Work out the finished part from the listing and answer in its coordinate system (mm). Face numbers are marked on the shaded views. A direction names the side the tool comes from. Round coordinates to 2 decimals unless told otherwise and drop trailing zeros. Order: outer loops, then holes, each group sorted by start corner. A loop starts at its lowest first (then second) coordinate and runs counter-clockwise, first axis right, second up. Notation, with made-up numbers: (89, -5.5) -> (114, -5.5) arc R20 cw to (114, 21.5) -> close; hole circle Ø9 at (-1, 7.25). An arc over 180 degrees is marked (long way). Use a Markdown table: item, result. Add a question column.
Item 1: Flat-ended cylindrical pins translate along their axes: P1, Ø5, axis at x = 77.5, y = -2, coming from the +Z side; P2, Ø20.5, axis at y = -24.5, z = 54.5, coming from the -X side; P3, Ø1.5, axis at y = -11.5, z = 29.5, coming from the +X side (3 decimals); P4, Ø2, axis at x = -40, y = 58.5, coming from the -Z side. Find the tip coordinate at first contact, or state that the pin passes through.
Item 2: A tool of negligible diameter and unlimited length cuts with its end or side. For the marked faces 1, 2, 3 and 4, from which of +Z, -Z, +X, -X, +Y, -Y can it reach the whole face along a straight path? Write none if from no direction.
Item 3: A cutting plane is placed at A-A, the plane x = 0. Determine the outline of the cut face in (y, z) (3 decimals).
Item 4: A cutting plane is placed at B-B, the plane z = 15. Determine the outline of the cut face in (x, y) (3 decimals).
Item 5: A cutting plane is placed at C-C, the plane y = 0. Determine the outline of the cut face in (x, z) (3 decimals), plus the area to 3 significant figures.
Item 6: For a pull along Y with two mould halves and no side action, classify the marked faces 5, 6, 7 and 8 as +Y half, -Y half, draft (parallel to the pull), parting line (faces both ways), or undercut.
Item 7: Find the intervals of material crossed by L1, parallel to Y at x = 0, z = 14 (3 decimals); L2, parallel to X at y = -3, z = 58; L3, parallel to Y at x = 115, z = 11, in increasing order. Write a range as [from, to].
Item 8: A cutting plane is placed at D-D, the plane x = 89.5. Determine the outline of the cut face in (y, z).
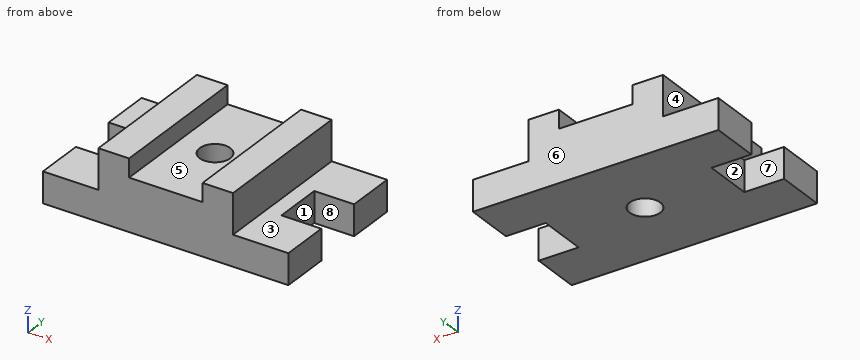
from build123d import *

# Parameters (mm, degrees)
F1_DEPTH  = 31.75
F2_W      = 69.6489959955
F2_H      = 152.4
F3_DEPTH  = 22.225
F4_W      = 31.5489959955
F4_H      = 152.4
F5_DEPTH  = 19.05
F6_W      = 31.5489959955
F6_H      = 31.75
F7_DEPTH  = 19.05
F9_D      = 31.75
F10_DEPTH = 19.05
F11_DEPTH = 19.05
F12_DEPTH = 19.05


# Not quite as in the source:
# - a feature names something its author has since deleted; it is built from what else it names


with BuildPart() as f1:
    # F0 (on Top) → F1 (new body)
    with BuildSketch(Plane.XY):
        Polygon((0, -76.2), (0, 76.2), (-127, 76.2), (-127, 25.4), (-85.725, 25.4), (-85.725, -25.4), (-127, -25.4), (-127, -76.2), align=None)
        Polygon((127, 25.4), (127, 76.2), (0, 76.2), (0, -76.2), (127, -76.2), (127, -25.4), (85.725, -25.4), (85.725, 25.4), align=None)
    extrude(amount=F1_DEPTH)

    # F2 (on face) → F3 (join)
    with BuildSketch(Plane.XY.offset(31.75)):
        with Locations((34.8244979978, 0)):
            Rectangle(F2_W, F2_H)
        with Locations((-34.8244979978, 0)):
            Rectangle(F2_W, F2_H)
    extrude(amount=F3_DEPTH)

    # F4 (on face) → F5 (join)
    with BuildSketch(Plane.XY.offset(53.975)):
        with Locations((53.8744979978, 0)):
            Rectangle(F4_W, F4_H)
    extrude(amount=F5_DEPTH)

    # F6 (on face) → F7 (join)
    with BuildSketch(Plane.XY):
        with Locations((53.8744979978, -60.325)):
            Rectangle(F6_W, F6_H)
        with Locations((-53.8744979978, -60.325)):
            Rectangle(F6_W, F6_H)
        with Locations((-53.8744979978, 60.325)):
            Rectangle(F6_W, F6_H)
        with Locations((53.8744979978, 60.325)):
            Rectangle(F6_W, F6_H)
    extrude(amount=F7_DEPTH)

    # F9 (through all)
    with Locations(Plane.XY.offset(53.975)):
        with Locations((0, 0)):
            Hole(F9_D / 2)

    # F6 (on face) → F10 (join)
    with BuildSketch(Plane.XY):
        with Locations((53.8744979978, 60.325)):
            Rectangle(F6_W, F6_H)
        with Locations((-53.8744979978, 60.325)):
            Rectangle(F6_W, F6_H)
        with Locations((-53.8744979978, -60.325)):
            Rectangle(F6_W, F6_H)
        with Locations((53.8744979978, -60.325)):
            Rectangle(F6_W, F6_H)
    extrude(amount=F10_DEPTH)

    # F4 (on face) → F11 (join)
    with BuildSketch(Plane.XY.offset(53.975)):
        with Locations((53.8744979978, 0)):
            Rectangle(F4_W, F4_H)
    extrude(amount=F11_DEPTH)

    # F4 (on face) → F12 (join)
    with BuildSketch(Plane.XY.offset(53.975)):
        Polygon((-37.8989959955, -76.2), (-37.8989959955, 76.2), (-69.6489959955, 76.2), (-69.6489959955, -76.2), (-38.1, -76.2), align=None)
    extrude(amount=F12_DEPTH)


solid = f1.part
Reported:
| question | item | result |
|---|---|---|
| 1 | P1 | z = 31.75 |
| 1 | P2 | x = -69.65 |
| 1 | P3 | x = 85.725 |
| 1 | P4 | z = 0 |
| 2 | face 1 | +Z, -Z, +X |
| 2 | face 2 | +Z, -Z, -X |
| 2 | face 3 | +Z, +X, +Y, -Y |
| 2 | face 4 | +Z, -X, +Y, -Y |
| 3 | outline | (-76.2, 0) -> (-15.875, 0) -> (-15.875, 53.975) -> (-76.2, 53.975) -> close; (15.875, 0) -> (76.2, 0) -> (76.2, 53.975) -> (15.875, 53.975) -> close |
| 4 | outline | (-127, -76.2) -> (127, -76.2) -> (127, -25.4) -> (85.725, -25.4) -> (85.725, 25.4) -> (127, 25.4) -> (127, 76.2) -> (-127, 76.2) -> (-127, 25.4) -> (-85.725, 25.4) -> (-85.725, -25.4) -> (-127, -25.4) -> close; hole circle Ø31.75 at (0, 0) |
| 5 | outline | (-85.725, 0) -> (-15.875, 0) -> (-15.875, 53.975) -> (-37.899, 53.975) -> (-37.899, 73.025) -> (-69.649, 73.025) -> (-69.649, 31.75) -> (-85.725, 31.75) -> close; (15.875, 0) -> (85.725, 0) -> (85.725, 31.75) -> (69.649, 31.75) -> (69.649, 73.025) -> (38.1, 73.025) -> (38.1, 53.975) -> (15.875, 53.975) -> close |
| 5 | area | 8,030 mm² |
| 6 | face 5 | draft |
| 6 | face 6 | +Y half |
| 6 | face 7 | undercut |
| 6 | face 8 | undercut |
| 7 | L1 | [-76.2, -15.875], [15.875, 76.2] |
| 7 | L2 | [-69.65, -37.9], [38.1, 69.65] |
| 7 | L3 | [-76.2, -25.4], [25.4, 76.2] |
| 8 | outline | (-76.2, 0) -> (-25.4, 0) -> (-25.4, 31.75) -> (-76.2, 31.75) -> close; (25.4, 0) -> (76.2, 0) -> (76.2, 31.75) -> (25.4, 31.75) -> close |
